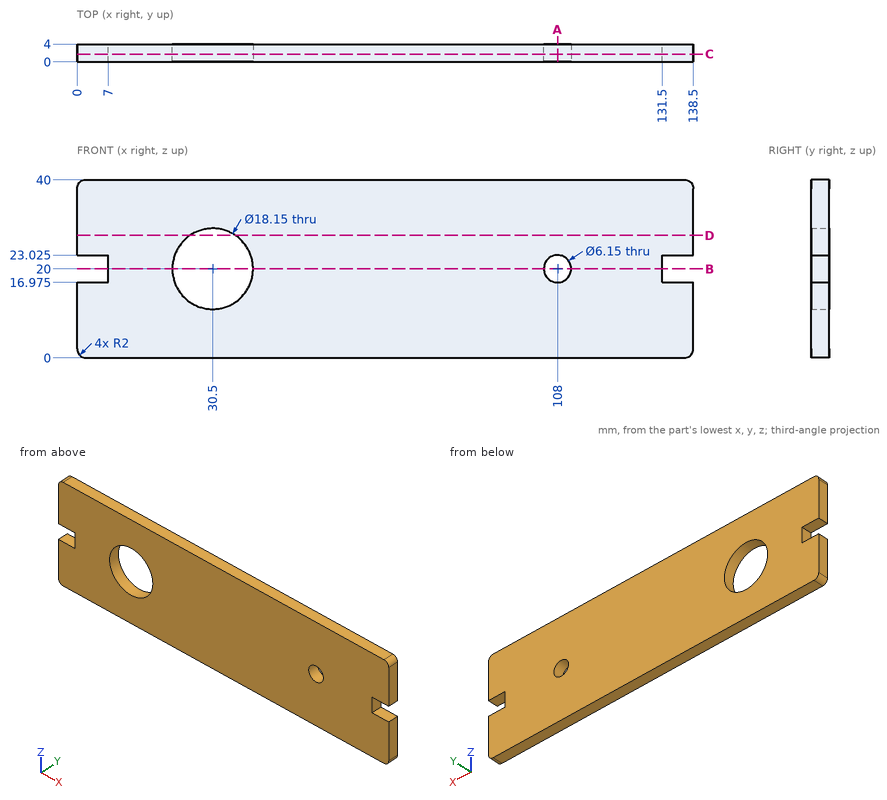
Geometry check sheet. Reference: drawing and pictorial views, mm from the part's lowest x, y, z. Round coordinates to 2 decimals unless told otherwise and drop trailing zeros. Loops run counter-clockwise (first coordinate to the right, second up) from the corner with the lowest first, then second, coordinate; pieces in that order, holes last.
1. Scan lines: probe 1 along Z at (x, y) = (108, 0.95) (3 decimals); probe 2 along X at (y, z) = (3.3, 18); probe 3 along Z at (x, y) = (31.5, 2). Record each from-to range of solid material in increasing order.
2. Sectioned sample at B-B on z = 20. Record the boundary of the cut face in (x, y) (3 decimals), and give its area (3 significant figures).
3. Sectioned sample at D-D on z = 27.5. Record the boundary of the cut face in (x, y), and give its area (3 significant figures).
4. Sectioned sample at C-C on y = 1.7. Record the boundary of the cut face in (x, z) (3 decimals).
5. Sectioned sample at A-A on x = 108. Record the boundary of the cut face in (y, z) (3 decimals).
Recorded:
1. probe 1: z = 0 to 16.925, 23.075 to 40
1. probe 2: x = 7 to 21.65, 39.35 to 105.66, 110.34 to 131.5
1. probe 3: z = 0 to 10.98, 29.02 to 40
2. outline: (7, 0) - (21.425, 0) - (21.425, 4) - (7, 4) - close; (39.575, 0) - (104.925, 0) - (104.925, 4) - (39.575, 4) - close; (111.075, 0) - (131.5, 0) - (131.5, 4) - (111.075, 4) - close
2. area: 401 mm2
3. outline: (0, 0) - (25.39, 0) - (25.39, 4) - (0, 4) - close; (35.61, 0) - (138.5, 0) - (138.5, 4) - (35.61, 4) - close
3. area: 513 mm2
4. outline: (0, 2) arc R2 ccw to (2, 0) - (136.5, 0) arc R2 ccw to (138.5, 2) - (138.5, 16.975) - (131.5, 16.975) - (131.5, 23.025) - (138.5, 23.025) - (138.5, 38) arc R2 ccw to (136.5, 40) - (2, 40) arc R2 ccw to (0, 38) - (0, 23.025) - (7, 23.025) - (7, 16.975) - (0, 16.975) - close; hole circle Ø18.15 at (30.5, 20); hole circle Ø6.15 at (108, 20)
5. outline: (0, 0) - (4, 0) - (4, 16.925) - (0, 16.925) - close; (0, 23.075) - (4, 23.075) - (4, 40) - (0, 40) - close
